from build123d import *

# Parameters (mm, degrees)
F0_R     = 5
F1_DEPTH = 75
F2_R     = 2.5
F3_DEPTH = 25
F4_R     = 2.5
F5_DEPTH = 20
F6_R     = 2.25
F7_DEPTH = 20
F8_R     = 2.5
F9_DEPTH = 25


with BuildPart() as f1:
    # F0 (on Front) → F1 (new body, symmetric)
    with BuildSketch(Plane.XZ):
        Circle(F0_R)
    extrude(amount=F1_DEPTH, both=True)

    # F2 (on face) → F3 (cut)
    with BuildSketch(Plane.XZ.offset(75)):
        Circle(F2_R)
    extrude(amount=-F3_DEPTH, mode=Mode.SUBTRACT)

    # F4 (on Right) → F5 (join)
    with BuildSketch(Plane.YZ):
        with Locations((21.7011971159, 0)):
            Circle(F4_R)
        with Locations((-22.3350814088, 0)):
            Circle(F4_R)
    extrude(amount=F5_DEPTH)

    # F6 (on face) → F7 (join)
    with BuildSketch(Plane(origin=(0, 75, 0), x_dir=(-1, 0, 0), z_dir=(0, 1, 0))):
        Circle(F6_R)
    extrude(amount=F7_DEPTH)

    # F8 (on Right) → F9 (join)
    with BuildSketch(Plane.YZ):
        with Locations((46.6944500804, 0)):
            Circle(F8_R)
        with Locations((-4.1080172062, 0)):
            Circle(F8_R)
        with Locations((-42.8937412798, 0)):
            Circle(F8_R)
    extrude(amount=-F9_DEPTH)


solid = f1.part
Model file for the job. Use its own axes, mm. A direction names the side the tool comes from. Give positions to 0.01 mm unless a question says otherwise; leave off trailing zeros. Order: outer loops, then holes, each group sorted by start corner. A loop starts at its lowest first (then second) coordinate and runs counter-clockwise, first axis right, second up. Notation, with made-up numbers: (32, 54) -> (68, 54) arc R30 ccw to (68, 86) -> close; hole circle Ø6 at (77, 34.25). An arc over 180 degrees is marked (long way). Use CSV: the item, a comma, the result in double quotes.
1. Drop flat-ended pins along their axis: pin 1 (5 mm diameter, centred on x = 3.5, y = -48, fed in from -Z); pin 2 (6 mm diameter, centred on x = 7, y = -14.5, fed in from +Z); pin 3 (1.5 mm diameter, centred on x = 0, z = -0.5, fed in from -Y). Give the stop position or say it passes through.
Outcome:
pin 1,"z = -4.9"
pin 2,"z = 3"
pin 3,"y = -50"
2. 3-axis set-ups, long thin cutter, end or side, ignore diameter. For faces 1 (the flat face through (2.2, 75, -1)), 2 (the cylindrical face through (-14.52, -1.723, 0.751)), 3 (the cylindrical face through (4.77, -1.05, 1.5)), 4 (the cylindrical face through (12.055, -24.833, 0.11)), 5 (the flat face through (0, 95, 0)): which of +Z, -Z, +X, -X, +Y, -Y reach the whole face in a straight line?
Outcome:
face 1,"+Y"
face 2,"-X"
face 3,"none"
face 4,"+X"
face 5,"+Z, -Z, +X, -X, +Y"
3. Band-saw the part on A-A, the plane x = -10.5. Give the cut face in (y, z), then the cut area to 3 significant figures.
Outcome:
outline,"circle Ø5 at (-42.89, 0); circle Ø5 at (-4.11, 0); circle Ø5 at (46.69, 0)"
area,"58.9 mm²"
4. Band-saw the part on D-D, the plane x = 14.5. Give the cut face in (y, z), then the cut area to 3 significant figures.
Outcome:
outline,"circle Ø5 at (-22.34, 0); circle Ø5 at (21.7, 0)"
area,"39.3 mm²"
5. Drill centre lines: line 1 along Z through (x, y) = (0, -67); line 2 along Y through (x, z) = (-13, 1.5); line 3 along Y through (x, z) = (-1, -4.25). Where is each one in solid material? Low to high. Write a range as from..to.
Outcome:
line 1,"-5..-2.5, 2.5..5"
line 2,"-44.89..-40.89, -6.11..-2.11, 44.69..48.69"
line 3,"-75..75"
6. Mould opens along Z. For faces 6 (the flat face through (-25, -43, 0)), 7 (the flat face through (0, -50, 0)), 8 (the cylindrical face through (-0.54, -62.68, -2.44)), 9 (the cylindrical face through (0.29, 84.86, 2.23)) say: +Z half, -Z half, draft (parallel to the pull), parting line (faces both ways), or undercut.
Outcome:
face 6,"draft"
face 7,"undercut"
face 8,"undercut"
face 9,"parting line"
7. Band-saw the part on C-C, the plane y = -64. Give the cut face in (x, z).
Outcome:
outline,"circle Ø10 at (0, 0); hole circle Ø5 at (0, 0)"
